```python
from build123d import *

# Parameters (mm, degrees)
BOSS_EXTRUDE1_START = -1.5875
SKETCH1_R           = 1.5875
BOSS_EXTRUDE1_DEPTH = 1.5875
BOSS_EXTRUDE2_START = 1.5875
SKETCH3_R           = 3.175
SKETCH3_R_2         = 1.5875
BOSS_EXTRUDE2_DEPTH = 1.5875
SKETCH4_R           = 3.175
SKETCH4_R_2         = 1.5875
BOSS_EXTRUDE3_DEPTH = 1.5875


with BuildPart() as part:
    # Sketch1 → Boss-Extrude1 (new body)
    with BuildSketch(Plane.XY.offset(BOSS_EXTRUDE1_START)):
        with BuildLine():
            Line((-40.989250829, -6.729951179), (-27.002785927, 32.342146276))
            ThreePointArc((-27.002785927, 32.342146276), (-22.943486276, 34.261348284), (-21.024284268, 30.202048634))
            Line((-21.024284268, 30.202048634), (-35.010749171, -8.870048821))
            ThreePointArc((-35.010749171, -8.870048821), (-39.070048821, -10.789250829), (-40.989250829, -6.729951179))
        make_face()
        with Locations((-24.013535097, 31.272097455)):
            Circle(SKETCH1_R, mode=Mode.SUBTRACT)
        with Locations((-38, -7.8)):
            Circle(SKETCH1_R, mode=Mode.SUBTRACT)
    extrude(amount=-BOSS_EXTRUDE1_DEPTH)

    # Sketch3 → Boss-Extrude2 (add)
    with BuildSketch(Plane.XY.offset(-1.5875).offset(BOSS_EXTRUDE2_START)):
        with Locations((-24.013535097, 31.272097455)):
            Circle(SKETCH3_R)
        with Locations((-24.013535097, 31.272097455)):
            Circle(SKETCH3_R_2, mode=Mode.SUBTRACT)
    extrude(amount=-BOSS_EXTRUDE2_DEPTH)

    # Sketch4 → Boss-Extrude3 (add)
    with BuildSketch(Plane(origin=(0, 0, -3.175), x_dir=(-1, 0, 0), z_dir=(0, 0, -1))):
        with Locations(Location((38, -7.8, 0), (0, 0, 199.69561783))):
            Circle(SKETCH4_R)
        with Locations(Location((38, -7.8, 0), (0, 0, 180))):
            Circle(SKETCH4_R_2, mode=Mode.SUBTRACT)
    extrude(amount=BOSS_EXTRUDE3_DEPTH)


solid = part.part
```
Here's how the part is built. I have some questions about the finished solid (model axes, mm). Coordinates: 2 decimals unless noted, no trailing zeros. Loops run counter-clockwise (first coordinate to the right, second up) from the corner with the lowest first, then second, coordinate; pieces in that order, holes last. Notation, with made-up numbers: (-16.75, -37.5) - (5.25, -37.5) arc R28 cw to (5.25, -15.5) - close; hole circle Ø5 at (56, 75). An arc over 180 degrees is marked (long way). Return JSON: item names as keys, results as strings. Group by question number.
Item 1: If we section it at B-B on x = -38: Write out the boundary of the cut face in (y, z) (1 decimal).
Item 2: I need wall thicknesses on line 1 (X direction, y = -7.8, z = -4.3) (1 decimal); line 2 (Z direction, x = -31.75, y = 3) (1 decimal); line 3 (X direction, y = -8, z = -1.65). Which ranges of each line are inside material? Lowest first, please. Write a range as from..to.
Item 3: If we section it at D-D on x = -33.25: Write out the boundary of the cut face in (y, z) (1 decimal).
Item 4: We'd pull the mould along Y, two halves only. Please class faces 1 (the face through (-34.094, 12.533, -2.37)), 2 (the face through (-23.16, 32.61, -1.57)), 3 (the face through (-30, 14, -3.175)): +Y half, -Y half, draft (parallel to the pull), parting line (faces both ways), or undercut.
Item 5: Will these pins go through, and if not, where does the flat tip stop? P1, Ø2, axis at y = 28, z = -3, coming from the -X side; P2, Ø6, axis at x = -30.5, y = 21, coming from the -Z side (3 decimals); P3, Ø10, axis at x = -37.5, y = 5, coming from the +Z side; P4, Ø2.5, axis at x = -24.01, y = 31.27, coming from the +Z side.
Calculated:
{
 "1": {"outline": "(-11, -4.8) - (-9.4, -4.8) - (-9.4, -1.6) - (-11, -1.6) - close; (-6.2, -4.8) - (-4.6, -4.8) - (-4.6, -3.2) - (1.6, -3.2) - (1.6, -1.6) - (-6.2, -1.6) - close"},
 "2": {"line 1": "x = -41.2..-39.6, -36.4..-34.8", "line 2": "z = -3.2..-1.6", "line 3": "x = -41.17..-39.57, -36.43..-34.7"},
 "3": {"outline": "(-4, -3.2) - (14.9, -3.2) - (14.9, -1.6) - (-4, -1.6) - close"},
 "4": {"face 1": "+Y half", "face 2": "undercut", "face 3": "draft"},
 "5": {"P1": "stops at x = -28.92", "P2": "stops at z = -3.175", "P3": "stops at z = -1.59", "P4": "passes through"}
}
